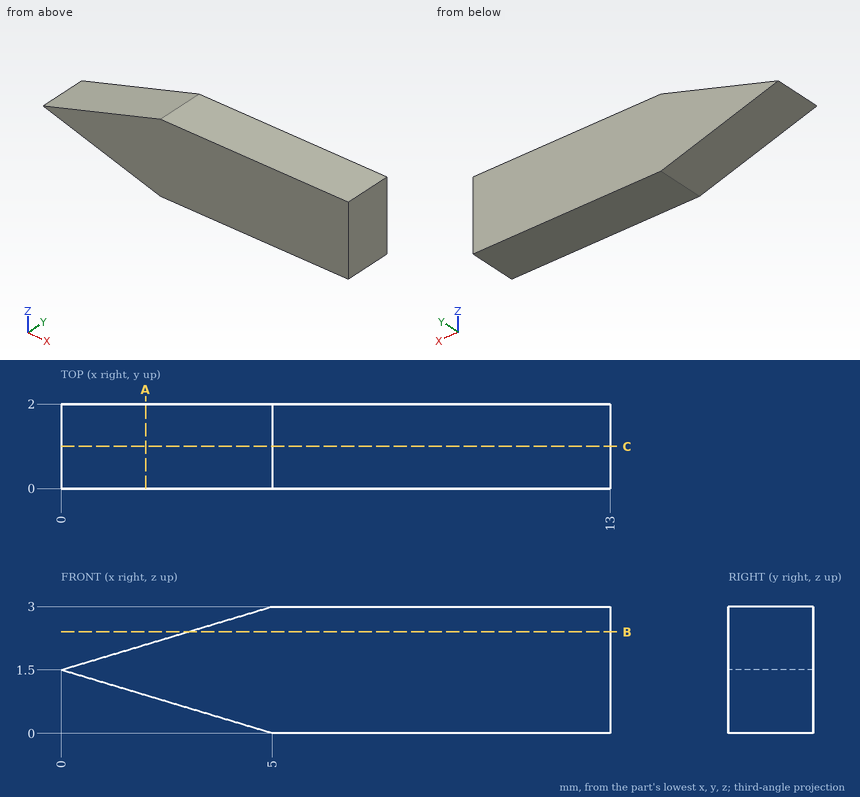
Geometry check sheet. Reference: drawing and pictorial views, mm from the part's lowest x, y, z. Give positions to 0.01 mm unless a question says otherwise; leave off trailing zeros. Order: outer loops, then holes, each group sorted by start corner. A loop starts at its lowest first (then second) coordinate and runs counter-clockwise, first axis right, second up. Notation, with made-up numbers: (40, -34) -> (83, -34) arc R10 ccw to (83, -15) -> close; hole circle Ø9 at (-30, 74). An arc over 180 degrees is marked (long way). Use CSV: the item, a comma, the result in double quotes. Start each with the question number.
1) Material ranges on line 1 (Z direction, x = 3.25, y = 1.4) (3 decimals); line 2 (Z direction, x = 1.25, y = 0.5) (3 decimals), recorded low to high. Write a range as from..to.
2) Sectioned sample at A-A, the plane x = 2. Record the boundary of the cut face in (y, z), plus the area to 3 significant figures.
3) Sectioned sample at C-C, the plane y = 1. Record the boundary of the cut face in (x, z), plus the area to 3 significant figures.
4) Sectioned sample at B-B, the plane z = 2.4. Record the boundary of the cut face in (x, y), plus the area to 3 significant figures.
Recorded:
1,line 1,"0.525..2.475"
1,line 2,"1.125..1.875"
2,outline,"(0, 0.9) -> (2, 0.9) -> (2, 2.1) -> (0, 2.1) -> close"
2,area,"2.40 mm2"
3,outline,"(0, 1.5) -> (5, 0) -> (13, 0) -> (13, 3) -> (5, 3) -> close"
3,area,"31.5 mm2"
4,outline,"(3, 0) -> (13, 0) -> (13, 2) -> (3, 2) -> close"
4,area,"20.0 mm2"
